The listing builds one solid part. Answer for the finished solid, in the listing's coordinates (mm). A direction names the side the tool comes from. Round coordinates to 2 decimals unless told otherwise and drop trailing zeros. Write each loop counter-clockwise with the first axis right and the second up, starting at its lowest first coordinate (ties: lowest second). Pieces come first, ordered by that corner, then holes.
Item 1: Find section A-A on z = 0. Give the vertices of the cut face in (x, y).
Item 2: A tool of negligible diameter and unlimited length cuts with its end or side. For faces 4 (the face through (7, -10, 0)), 5 (the face through (-11.45, 0.14, -13.646)), from which of +Z, -Z, +X, -X, +Y, -Y can it reach the whole face along a straight path? Write none if from no direction.
Item 3: Find section B-B on y = 4.75. Give the number of separate pieces and of enclosed holes in the cut face, then the cut area to 3 significant figures.
Item 4: Find section D-D on z = 25. Give the vertices of the cut face in (x, y).
Item 5: Find the intervals of material crossed by probe 1 along Z at (x, y) = (1.5, -2.25) (3 decimals); probe 2 along Z at (x, y) = (-5, 4.5); probe 3 along X at (y, z) = (6.25, 18.5), in increasing order.
Item 6: Find section C-C on x = 0. Give the vertices of the cut face in (y, z).
Item 7: For a pull along Z with two mould halves and no side action, classify faces 1 (the face through (2.6, 13, 7.2)), 2 (the face through (33.71, 0.14, -4.43)), 3 (the face through (28, 0, 0)) as +Z half, -Z half, draft (parallel to the pull), parting line (faces both ways), or undercut.
Item 8: Each of these flat-tipped pins is pushed along its axis until it touches: pin 1 (3 mm diameter, centred on y = 5.5, z = 0.5, fed in from -X); pin 2 (8 mm diameter, centred on y = 1.5, z = -27, fed in from -X); pin 3 (3 mm diameter, centred on x = -16.5, z = 23, fed in from +Y); pin 4 (8 mm diameter, centred on x = 2, y = 2, fed in from -Z). Where does it stop, or does it pass through?
```python
from build123d import *

# Parameters (mm, degrees)
SKETCH_1_R          = 34
SKETCH_1_R_2        = 11
EXTRUDE_1_DEPTH     = 10
SKETCH_1_3_R        = 11
SKETCH_1_3_R_2      = 7.5
EXTRUDE_2_DEPTH     = 13
SKETCH_1_4_R        = 7.5
SKETCH_1_4_R_2      = 2.7
EXTRUDE_3_DEPTH     = 15
EXTRUDE_START       = -10
SKETCH_1_6_R        = 11
SKETCH_1_6_R_2      = 7.5
SKETCH_1_6_R_3      = 2.7
EXTRUDE_4_DEPTH     = 10
CUT_EXTRUDE_1_DEPTH = 53.076866265


with BuildPart() as part:
    # 草图1 → 凸台-拉伸1 (new, symmetric)
    with BuildSketch(Plane(origin=(0, 0, 0), x_dir=(1, 0, 0), z_dir=(0, 1, 0))):
        with Locations(Location((0, 0, 0), (0, 0, 270))):
            Circle(SKETCH_1_R)
        with Locations(Location((0, 0, 0), (0, 0, 270))):
            Circle(SKETCH_1_R_2, mode=Mode.SUBTRACT)
    extrude(amount=EXTRUDE_1_DEPTH, both=True)

    # 草图1<3> → 凸台-拉伸2 (add)
    with BuildSketch(Plane(origin=(0, 0, 0), x_dir=(1, 0, 0), z_dir=(0, 1, 0))):
        with Locations(Location((0, 0, 0), (0, 0, 270))):
            Circle(SKETCH_1_3_R)
        with Locations(Location((0, 0, 0), (0, 0, 90))):
            Circle(SKETCH_1_3_R_2, mode=Mode.SUBTRACT)
    extrude(amount=EXTRUDE_2_DEPTH)

    # 草图1<4> → 凸台-拉伸3 (add)
    # profile 1 of 3: a face of its own
    with BuildSketch(Plane(origin=(0, 0, 0), x_dir=(1, 0, 0), z_dir=(0, 1, 0))):
        with Locations(Location((0, 0, 0), (0, 0, 270))):
            Circle(SKETCH_1_4_R)
        Circle(SKETCH_1_4_R_2, mode=Mode.SUBTRACT)
    # profile 2 of 3: a face of its own
    with BuildSketch(Plane(origin=(0, 0, 0), x_dir=(1, 0, 0), z_dir=(0, 1, 0))):
        with BuildLine():
            ThreePointArc((2.7, 0), (2.478406746, 1.071214264), (1.85, 1.966596044))
            Line((1.85, 1.966596044), (1.85, -1.966596044))
            ThreePointArc((1.85, -1.966596044), (2.478406746, -1.071214264), (2.7, 0))
        make_face()
    # profile 3 of 3: a face of its own
    with BuildSketch(Plane(origin=(0, 0, 0), x_dir=(1, 0, 0), z_dir=(0, 1, 0))):
        with BuildLine():
            Line((-1.85, -1.966596044), (-1.85, 1.966596044))
            ThreePointArc((-1.85, 1.966596044), (-2.7, 0), (-1.85, -1.966596044))
        make_face()
    extrude(amount=EXTRUDE_3_DEPTH)

    # 草图1<6> → 凸台-拉伸4 (add)
    # profile 1 of 4: a face of its own
    with BuildSketch(Plane(origin=(0, 0, 0), x_dir=(1, 0, 0), z_dir=(0, 1, 0)).offset(EXTRUDE_START)):
        with Locations(Location((0, 0, 0), (0, 0, 90))):
            Circle(SKETCH_1_6_R)
        with Locations(Location((0, 0, 0), (0, 0, 270))):
            Circle(SKETCH_1_6_R_2, mode=Mode.SUBTRACT)
    # profile 2 of 4: a face of its own
    with BuildSketch(Plane(origin=(0, 0, 0), x_dir=(1, 0, 0), z_dir=(0, 1, 0)).offset(EXTRUDE_START)):
        with Locations(Location((0, 0, 0), (0, 0, 270))):
            Circle(SKETCH_1_6_R_2)
        Circle(SKETCH_1_6_R_3, mode=Mode.SUBTRACT)
    # profile 3 of 4: a face of its own
    with BuildSketch(Plane(origin=(0, 0, 0), x_dir=(1, 0, 0), z_dir=(0, 1, 0)).offset(EXTRUDE_START)):
        with BuildLine():
            Line((-1.85, -1.966596044), (-1.85, 1.966596044))
            ThreePointArc((-1.85, 1.966596044), (-2.7, 0), (-1.85, -1.966596044))
        make_face()
    # profile 4 of 4: a face of its own
    with BuildSketch(Plane(origin=(0, 0, 0), x_dir=(1, 0, 0), z_dir=(0, 1, 0)).offset(EXTRUDE_START)):
        with BuildLine():
            ThreePointArc((2.7, 0), (2.478406746, 1.071214264), (1.85, 1.966596044))
            Line((1.85, 1.966596044), (1.85, -1.966596044))
            ThreePointArc((1.85, -1.966596044), (2.478406746, -1.071214264), (2.7, 0))
        make_face()
    extrude(amount=EXTRUDE_4_DEPTH)

    # 草图2 → 切除-拉伸1 (cut, through all)
    with BuildSketch(Plane(origin=(0, 10, 0), x_dir=(1, 0, 0), z_dir=(0, 1, 0))):
        with BuildLine():
            Line((-7.070663707, 8.426488874), (-15.95356892, 19.012723075))
            ThreePointArc((-15.95356892, 19.012723075), (-16.62289939, 21.381720221), (-15.294087861, 23.454016212))
            ThreePointArc((-15.294087861, 23.454016212), (0, 28), (15.294087861, 23.454016212))
            ThreePointArc((15.294087861, 23.454016212), (16.62289939, 21.381720221), (15.95356892, 19.012723075))
            Line((15.95356892, 19.012723075), (7.070663707, 8.426488874))
            ThreePointArc((7.070663707, 8.426488874), (0, 11), (-7.070663707, 8.426488874))
        make_face()
        with BuildLine():
            Line((8.426488874, -7.070663707), (19.012723075, -15.95356892))
            ThreePointArc((19.012723075, -15.95356892), (21.381720221, -16.62289939), (23.454016212, -15.294087861))
            ThreePointArc((23.454016212, -15.294087861), (28, 0), (23.454016212, 15.294087861))
            ThreePointArc((23.454016212, 15.294087861), (21.381720221, 16.62289939), (19.012723075, 15.95356892))
            Line((19.012723075, 15.95356892), (8.426488874, 7.070663707))
            ThreePointArc((8.426488874, 7.070663707), (11, 0), (8.426488874, -7.070663707))
        make_face()
        with BuildLine():
            Line((-7.070663707, -8.426488874), (-15.95356892, -19.012723075))
            ThreePointArc((-15.95356892, -19.012723075), (-16.62289939, -21.381720221), (-15.294087861, -23.454016212))
            ThreePointArc((-15.294087861, -23.454016212), (0, -28), (15.294087861, -23.454016212))
            ThreePointArc((15.294087861, -23.454016212), (16.62289939, -21.381720221), (15.95356892, -19.012723075))
            Line((15.95356892, -19.012723075), (7.070663707, -8.426488874))
            ThreePointArc((7.070663707, -8.426488874), (0, -11), (-7.070663707, -8.426488874))
        make_face()
        with BuildLine():
            Line((-8.426488874, 7.070663707), (-19.012723075, 15.95356892))
            ThreePointArc((-19.012723075, 15.95356892), (-21.381720221, 16.62289939), (-23.454016212, 15.294087861))
            ThreePointArc((-23.454016212, 15.294087861), (-28, 0), (-23.454016212, -15.294087861))
            ThreePointArc((-23.454016212, -15.294087861), (-21.381720221, -16.62289939), (-19.012723075, -15.95356892))
            Line((-19.012723075, -15.95356892), (-8.426488874, -7.070663707))
            ThreePointArc((-8.426488874, -7.070663707), (-11, 0), (-8.426488874, 7.070663707))
        make_face()
    extrude(amount=-CUT_EXTRUDE_1_DEPTH, mode=Mode.SUBTRACT)


solid = part.part
```
Check values:
1. outline: (-34, -10) - (-28, -10) - (-28, 10) - (-34, 10) - close; (-11, -10) - (-1.85, -10) - (-1.85, 15) - (-7.5, 15) - (-7.5, 13) - (-11, 13) - close; (1.85, -10) - (11, -10) - (11, 13) - (7.5, 13) - (7.5, 15) - (1.85, 15) - close; (28, -10) - (34, -10) - (34, 10) - (28, 10) - close
2. face 4: +Z, -Z, +X, -X, -Y
2. face 5: +Y, -Y
3. separate pieces: 1
3. enclosed holes: 5
3. area: 1,780 mm2
4. outline: (-23.04, -10) - (-12.61, -10) - (-12.61, 10) - (-23.04, 10) - close; (12.61, -10) - (23.04, -10) - (23.04, 10) - (12.61, 10) - close
5. probe 1: z = -33.967 to -27.96, -10.897 to -2.245, 2.245 to 10.897, 27.96 to 33.967
5. probe 2: z = -33.63 to -27.55, -9.8 to 9.8, 27.55 to 33.63
5. probe 3: x = -28.53 to -15.52, 15.52 to 28.53
6. outline: (-10, -34) - (10, -34) - (10, -28) - (-10, -28) - close; (-10, -11) - (13, -11) - (13, -7.5) - (15, -7.5) - (15, -2.7) - (-10, -2.7) - close; (-10, 2.7) - (15, 2.7) - (15, 7.5) - (13, 7.5) - (13, 11) - (-10, 11) - close; (-10, 28) - (10, 28) - (10, 34) - (-10, 34) - close
7. face 1: draft
7. face 2: parting line
7. face 3: undercut
8. pin 1: stops at x = -34
8. pin 2: stops at x = -25.04
8. pin 3: stops at y = 10
8. pin 4: stops at z = -34
